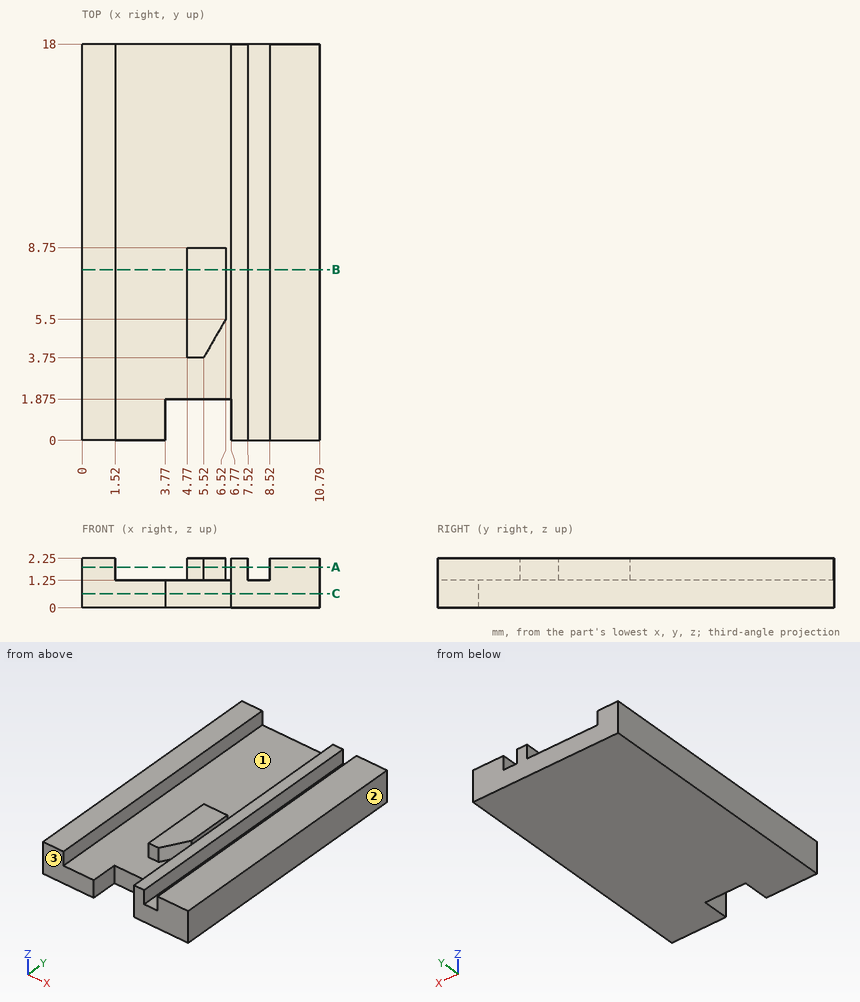
Could you check a few things on this drawing? It's one solid part, dimensions in mm from its lowest x, y, z. Give positions to 0.01 mm unless a question says otherwise; leave off trailing zeros. Write each loop counter-clockwise with the first axis right and the second up, starting at its lowest first coordinate (ties: lowest second). Pieces come first, ordered by that corner, then holes. Notation, with made-up numbers: (55.25, -26.75) -> (76.25, -26.75) arc R13 ccw to (76.25, -20.75) -> close; hole circle Ø5 at (86.25, 71.5). An arc over 180 degrees is marked (long way). Answer as a JSON object with one key per item and string values.
Q1. We'd pull the mould along X, two halves only. Please class the marked faces 1, 2 and 3: released by +X, released by -X, zero draft, split by the parting line, or undercut.
Taken from the geometry:
{"face 1": "undercut", "face 2": "released by +X", "face 3": "zero draft"}
Q2. Will this pin go through, and if not, where does the flat tip stop? pin 1 Ø0.6 at (x, z) = (5.5, 1.5) entering from -Y (3 decimals).
Taken from the geometry:
{"pin 1": "stops at y = 1.875"}
Q3. Please list where these lines run through material, in increasing order: L1, parallel to X at y = 11.25, z = 1.65; L2, parallel to X at y = 8.25, z = 2.1; L3, parallel to Z at x = 4.5, y = 12.25.
Taken from the geometry:
{"L1": "x = 0 to 1.52, 6.77 to 7.52, 8.52 to 10.79", "L2": "x = 0 to 1.52, 4.77 to 6.52, 6.77 to 7.52, 8.52 to 10.79", "L3": "z = 0 to 1.25"}
Q4. Suppose I cut it at C-C on z = 0.65. Write out the boundary of the cut face in (x, y) (3 decimals).
Taken from the geometry:
{"outline": "(0, 0) -> (3.77, 0) -> (3.77, 1.875) -> (6.77, 1.875) -> (6.77, 0) -> (10.79, 0) -> (10.79, 18) -> (0, 18) -> close"}
Q5. Suppose I cut it at A-A on z = 1.85. Write out the boundary of the cut face in (x, y), then the cut area to 3 significant figures.
Taken from the geometry:
{"outline": "(0, 0) -> (1.52, 0) -> (1.52, 18) -> (0, 18) -> close; (4.77, 3.75) -> (5.52, 3.75) -> (6.52, 5.5) -> (6.52, 8.75) -> (4.77, 8.75) -> close; (6.77, 0) -> (7.52, 0) -> (7.52, 18) -> (6.77, 18) -> close; (8.52, 0) -> (10.79, 0) -> (10.79, 18) -> (8.52, 18) -> close", "area": "89.6 mm²"}
Q6. Suppose I cut it at B-B on y = 7.75. Write out the boundary of the cut face in (x, z), then the cut area to 3 significant figures.
Taken from the geometry:
{"outline": "(0, 0) -> (10.79, 0) -> (10.79, 2.25) -> (8.52, 2.25) -> (8.52, 1.25) -> (7.52, 1.25) -> (7.52, 2.25) -> (6.77, 2.25) -> (6.77, 1.25) -> (6.52, 1.25) -> (6.52, 2.25) -> (4.77, 2.25) -> (4.77, 1.25) -> (1.52, 1.25) -> (1.52, 2.25) -> (0, 2.25) -> close", "area": "19.8 mm²"}
